```python
from build123d import *

# Parameters (mm, degrees)
SKETCH2_R           = 27
BOSS_EXTRUDE1_DEPTH = 10
BOSS_EXTRUDE2_DEPTH = 10
FILLET1_R           = 10


with BuildPart() as part:
    # Sketch2 → Boss-Extrude1 (new body)
    with BuildSketch(Plane(origin=(0, 0, 0), x_dir=(1, 0, 0), z_dir=(0, 1, 0))):
        with Locations(Location((0, 0, 0), (0, 0, 270))):
            Circle(SKETCH2_R)
    extrude(amount=BOSS_EXTRUDE1_DEPTH)

    # Sketch3 → Boss-Extrude2 (add, symmetric)
    with BuildSketch(Plane(origin=(0, 0, 0), x_dir=(0, 0, -1), z_dir=(1, 0, 0))):
        with BuildLine():
            Line((27, 10), (-27, 10))
            Line((-27, 10), (-27, 98))
            Line((-27, 98), (-51.368939129, 143.705592112))
            ThreePointArc((-51.368939129, 143.705592112), (-54.192675617, 153.062397712), (-53.213203436, 162.786796564))
            Line((-53.213203436, 162.786796564), (-32, 184))
            Line((-32, 184), (-32, 199))
            Line((-32, 199), (-27, 199))
            Line((-27, 199), (-27, 179))
            Line((-27, 179), (-48.213203436, 157.786796564))
            Line((-48.213203436, 157.786796564), (-27, 118))
            Line((-27, 118), (27, 118))
            Line((27, 118), (48.213203436, 157.786796564))
            Line((48.213203436, 157.786796564), (27, 179))
            Line((27, 179), (27, 199))
            Line((27, 199), (32, 199))
            Line((32, 199), (32, 184))
            Line((32, 184), (53.213203436, 162.786796564))
            ThreePointArc((53.213203436, 162.786796564), (54.192675617, 153.062397712), (51.368939129, 143.705592112))
            Line((51.368939129, 143.705592112), (27, 98))
            Line((27, 98), (27, 10))
        make_face()
    extrude(amount=BOSS_EXTRUDE2_DEPTH, both=True)

    # Fillet1
    fillet1_edges = [part.edges().sort_by_distance(p)[0] for p in [
        (0, 157.786796564, -48.213203436),
        (0, 118, -27),
        (0, 118, 27),
        (0, 157.786796564, 48.213203436),
    ]]
    fillet(fillet1_edges, radius=FILLET1_R)


solid = part.part
```
Check sheet for the modelled part. Datum: model origin and axes. Units: mm. A direction names the side the tool comes from. Round coordinates to 2 decimals unless told otherwise and drop trailing zeros. Loops run counter-clockwise (first coordinate to the right, second up) from the corner with the lowest first, then second, coordinate; pieces in that order, holes last. Notation, with made-up numbers: (69.5, 89.5) - (109.5, 89.5) arc R25 ccw to (109.5, 101.5) - close; hole circle Ø8 at (42.25, 62.25). An arc over 180 degrees is marked (long way). Answer as a JSON object with one key per item and string values. Group by question number.
Q1. Scan lines: line 1 along Z through (x, y) = (-9, 57); line 2 along Y through (x, z) = (-21.5, -8.5); line 3 along X through (y, z) = (68, 2). Record each from-to range of solid material in increasing order. Write a range as [from, to].
Q2. Gauge pin test, flat ends, axial feed: P1, Ø6, axis at x = -2.5, y = 190, coming from the +Z side; P2, Ø1.5, axis at x = 16.5, z = -19.5, coming from the +Y side; P3, Ø16, axis at x = 2, z = 5.5, coming from the +Y side; P4, Ø2, axis at x = 6, z = 25.5, coming from the -Y side. Record the tip position at first contact, or that the pin passes through.
Q3. Mould release check, pull along Z, two halves, no side actions. Record for faces 6 (the face through (0.14, 137.47, 37.38)), 7 (the face through (0.14, 120.533, 39.014)), 8 (the face through (10, 84, -4)), 9 (the face through (0, 192, -32)): released by +Z, released by -Z, zero draft, split by the parting line, or undercut.
Q4. Sectioned sample at C-C, the plane z = 40.5. Enter the section's corners in (x, y), plus the area to 3 significant figures.
Q5. Sectioned sample at A-A, the plane z = 0. Enter the section's corners in (x, y).
Q6. Set-up check for faces 1 (the face through (0, 191, 32)), 2 (the face through (-16, 10, 0)), 3 (the face through (0, 171, -35)), 4 (the face through (0, 53, 27)), 5 (the face through (17, 10, 0)): record each of +Z, -Z, +X, -X, +Y, -Y from which the full face is reachable in a straight line by a thin tool's end or side.
Q7. Sectioned sample at D-D, the plane y = 76.5. Enter the section's corners in (x, z), plus the area to 3 significant figures.
Q8. Sectioned sample at B-B, the plane x = -6. Enter the section's corners in (y, z).
Solution:
{
 "1": {"line 1": "z = [-27, 27]", "line 2": "y = [0, 10]", "line 3": "x = [-10, 10]"},
 "2": {"P1": "stops at z = 32", "P2": "stops at y = 10", "P3": "stops at y = 118", "P4": "stops at y = 0"},
 "3": {"face 6": "undercut", "face 7": "released by +Z", "face 8": "zero draft", "face 9": "released by -Z"},
 "4": {"outline": "(-10, 123.32) - (10, 123.32) - (10, 143.32) - (-10, 143.32) - close; (-10, 165.5) - (10, 165.5) - (10, 175.5) - (-10, 175.5) - close", "area": "600 mm²"},
 "5": {"outline": "(-27, 0) - (27, 0) - (27, 10) - (10, 10) - (10, 118) - (-10, 118) - (-10, 10) - (-27, 10) - close"},
 "6": {"face 1": "+Z, +X, -X, +Y", "face 2": "+Z, -Z, -X, +Y", "face 3": "+X, -X", "face 4": "+Z, +X, -X, -Y", "face 5": "+Z, -Z, +X, +Y"},
 "7": {"outline": "(-10, -27) - (10, -27) - (10, 27) - (-10, 27) - close", "area": "1,080 mm²"},
 "8": {"outline": "(0, -26.32) - (10, -26.32) - (10, -27) - (98, -27) - (143.71, -51.37) arc R25 ccw to (162.79, -53.21) - (184, -32) - (199, -32) - (199, -27) - (179, -27) - (163.03, -42.97) arc R10 cw to (151.25, -44.73) - (123.3, -29.82) arc R10 cw to (118, -21) - (118, 21) arc R10 cw to (123.3, 29.82) - (151.25, 44.73) arc R10 cw to (163.03, 42.97) - (179, 27) - (199, 27) - (199, 32) - (184, 32) - (162.79, 53.21) arc R25 ccw to (143.71, 51.37) - (98, 27) - (10, 27) - (10, 26.32) - (0, 26.32) - close"}
}
